Geometry check sheet. Reference: the model listing, model coordinates, mm. Face numbers are marked on the shaded views. A direction names the side the tool comes from. Coordinates: 2 decimals unless noted, no trailing zeros. Loops run counter-clockwise (first coordinate to the right, second up) from the corner with the lowest first, then second, coordinate; pieces in that order, holes last. Notation, with made-up numbers: (-32.75, 19.25) - (-7.75, 19.25) arc R31 ccw to (-7.75, 55.25) - close; hole circle Ø2 at (67.5, 70). An arc over 180 degrees is marked (long way). Write each question's results on one line, items separated by ' | '. Start each with the question number.
(1) Go/stop test with flat-tipped pins: pin 1 Ø6.5 at (x, y) = (-15, 20) entering from +Z; pin 2 Ø12 at (x, y) = (-16.5, 16) entering from -Z; pin 3 Ø12 at (y, z) = (8.5, 39.5) entering from +X; pin 4 Ø10 at (x, z) = (-5.5, 41) entering from +Y. Record where each tip stops, or that it passes through.
(2) Sectioned sample at C-C (y = 16). Enter the section's corners in (x, z), plus the area to 3 significant figures.
(3) Mould release check, pull along Z, two halves, no side actions. Record for the marked faces 4, 5 and 6: pulls with the +Z half, pulls with the -Z half, needs draft (parallel to the pull), parting line crosses it, or undercut.
(4) Material ranges on probe 1 along Z at (x, y) = (-5, 10); probe 2 along Y at (x, z) = (-15, 5.2); probe 3 along Z at (x, y) = (-6, 2.1), recorded low to high.
(5) Sectioned sample at B-B (z = 30). Enter the section's corners in (x, y), plus the area to 3 significant figures.
(6) Sectioned sample at D-D (z = 54.5). Enter the section's corners in (x, y).
(7) Sectioned sample at A-A (y = 20). Enter the section's corners in (x, z).
(8) Access from +Z, -Z, +X, -X, +Y, -Y to the whole of each face (thin tool, end or side, straight path). Record for the marked faces 1, 2 and 3.
Autodesk Inventor part; units mm, degrees
ref_plane "YZ Plane" through (0, 0, 0) normal (1, 0, 0) x (0, 1, 0)
ref_plane "XZ Plane" through (0, 0, 0) normal (0, 1, 0) x (-1, 0, 0)
ref_plane "XY Plane" through (0, 0, 0) normal (0, 0, 1) x (1, 0, 0)
sketch "Sketch1" plane through (0, 0, 0) normal (0, 1, 0) x (-1, 0, 0)
  line L0 (0, 0) -> (24, 0)
  line L1 (24, 0) -> (24, 60)
  line L2 (24, 60) -> (0, 60)
  line L3 (0, 60) -> (0, 0)
  line L4 (24, 30) -> (0, 30) construction
  circle A0 centre (18, 30) radius 2.6
  circle A1 centre (6, 30) radius 2.6
  dimension "d0" = 24
  dimension "d1" = 60
  dimension "d2" = 5.2
  dimension "d3" = 5.2
  dimension "d4" = 6
  dimension "d5" = 6
  dimension "d6" = 12
extrude "Extrusion1" add sketch "Sketch1" along normal blind 6
sketch "Sketch2" plane through (0, 6, 0) normal (0, 1, 0) x (1, 0, 0)
  line L0 (-24, 0) -> (-24, -60)
  line L1 (-24, -4.5) -> (0, -4.5)
  line L2 (0, -4.5) -> (0, -8)
  line L3 (0, -8) -> (-24, -8)
  line L4 (-24, -8) -> (-24, -4.5)
  line L5 (-24, -55.5) -> (0, -55.5)
  line L6 (0, -55.5) -> (0, -52)
  line L7 (0, -52) -> (-24, -52)
  line L8 (-24, -52) -> (-24, -55.5)
  line L9 (0, 0) -> (-24, 0)
  dimension "d9" = 24
  dimension "d10" = 24
  dimension "d12" = 51
  dimension "d13" = 3.5
  dimension "d14" = 3.5
  dimension "d15" = 4.5
extrude "Extrusion2" add sketch "Sketch2" along normal blind 30
sketch "Sketch3" plane through (-24, 6, 55.5) normal (0, 0, 1) x (1, 0, 0)
  point P0 (24, -6)
sketch "Sketch4" plane through (-24, 6, 55.5) normal (0, 0, 1) x (1, 0, 0)
  circle A0 centre (9, 14) radius 2.75
  line L0 (0, 0) -> (24, 0)
  line L1 (0, 0) -> (0, 30)
  point P0 (24, -6)
  dimension "d18" = 5.5
  dimension "d19" = 14
  dimension "d20" = 9
extrude "Extrusion3" cut sketch "Sketch4" against normal through all
fillet "Fillet1" radius 12 2 edges at (0, 36, 53.75) (0, 36, 6.25)
fillet "Fillet2" radius 6 2 edges at (-24, 36, 53.75) (-24, 36, 6.25)
equation "\"d5\" = d4"
equation "\"d14\" = d13"
properties part number "X Axis Drag Chain Mount Statonary Bolted"
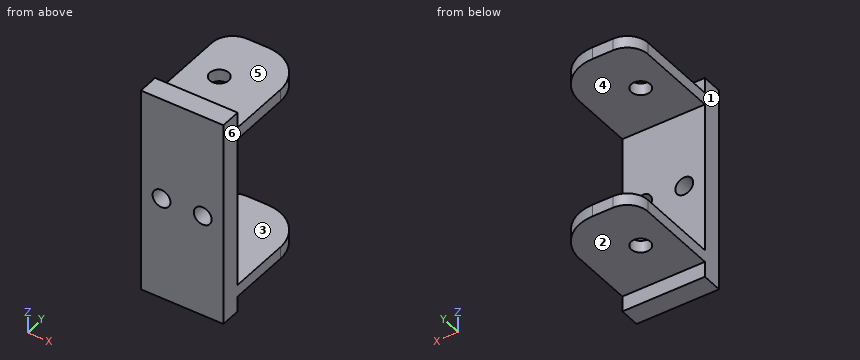
Outcome:
1) pin 1: stops at z = 55.5 | pin 2: stops at z = 4.5 | pin 3: stops at x = 0 | pin 4: stops at y = 6
2) outline: (-24, 4.5) - (0, 4.5) - (0, 8) - (-24, 8) - close; (-24, 52) - (0, 52) - (0, 55.5) - (-24, 55.5) - close | area: 168 mm2
3) face 4: undercut | face 5: pulls with the +Z half | face 6: needs draft
4) probe 1: z = 4.5 to 8, 52 to 55.5 | probe 2: y = 0 to 17.25, 22.75 to 36 | probe 3: z = 0 to 27.4, 32.6 to 60
5) outline: (-24, 0) - (-20.6, 0) - (-20.6, 6) - (-24, 6) - close; (-15.4, 0) - (-8.6, 0) - (-8.6, 6) - (-15.4, 6) - close; (-3.4, 0) - (0, 0) - (0, 6) - (-3.4, 6) - close | area: 81.6 mm2
6) outline: (-24, 0) - (0, 0) - (0, 24) arc R12 ccw to (-12, 36) - (-18, 36) arc R6 ccw to (-24, 30) - close; hole circle Ø5.5 at (-15, 20)
7) outline: (-24, 4.5) - (-17.75, 4.5) - (-17.75, 8) - (-24, 8) - close; (-24, 52) - (-17.75, 52) - (-17.75, 55.5) - (-24, 55.5) - close; (-12.25, 4.5) - (0, 4.5) - (0, 8) - (-12.25, 8) - close; (-12.25, 52) - (0, 52) - (0, 55.5) - (-12.25, 55.5) - close
8) face 1: +Z, -Z, -X, +Y, -Y | face 2: -Z, +X, -X, +Y | face 3: +X, -X, +Y
